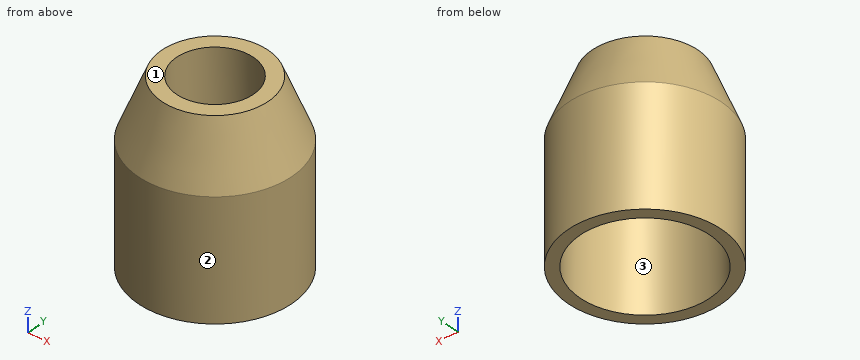
```python
from build123d import *

# Parameters (mm, degrees)
SKETCH177_R     = 6.5
PAD072_DEPTH    = 20
SKETCH178_R     = 3.25
POCKET069_DEPTH = 20.001
SKETCH179_R     = 5.5
POCKET070_DEPTH = 15
SKETCH180_W     = 0.76168
SKETCH180_H     = 6.5
PAD073_DEPTH    = 2
SKETCH182_W     = 6.5
SKETCH182_H     = 2
POCKET071_DEPTH = 6.501
SKETCH183_R     = 7.331051
POCKET072_DEPTH = 5


with BuildPart() as part:
    # Sketch177 → Pad072 (new body)
    with BuildSketch(Plane.XY):
        Circle(SKETCH177_R)
    extrude(amount=PAD072_DEPTH)

    # Sketch178 (on Face3 of Pad072) → Pocket069 (cut, through all)
    with BuildSketch(Plane.XY.offset(20)):
        Circle(SKETCH178_R)
    extrude(amount=-POCKET069_DEPTH, mode=Mode.SUBTRACT)

    # Sketch179 (on Face2 of Pocket069) → Pocket070 (cut)
    with BuildSketch(Plane(origin=(0, 0, 0), x_dir=(1, 0, 0), z_dir=(0, 0, -1))):
        Circle(SKETCH179_R)
    extrude(amount=-POCKET070_DEPTH, mode=Mode.SUBTRACT)

    # Sketch180 (on Face3 of Pocket070) → Pad073 (join)
    with BuildSketch(Plane.XY.offset(20)):
        with Locations((0.38084, -3.25)):
            Rectangle(SKETCH180_W, SKETCH180_H)
    extrude(amount=PAD073_DEPTH)

    # Sketch181 (on Face9 of Pad073) → Groove001 (revolve, cut)
    with BuildSketch(Plane(origin=(0, 0, 0), x_dir=(0, -1, 0), z_dir=(-1, 0, 0))):
        Polygon((4.5, 20), (6.5, 20), (6.5, 15), align=None)
    revolve(axis=Axis((0, 0, 0), (0, 0, 1)), mode=Mode.SUBTRACT)

    # Sketch182 (on Face9 of Groove001) → Pocket071 (cut, through all)
    with BuildSketch(Plane(origin=(0, 0, 0), x_dir=(0, -1, 0), z_dir=(-1, 0, 0))):
        with Locations((3.25, 21)):
            Rectangle(SKETCH182_W, SKETCH182_H)
    extrude(amount=-POCKET071_DEPTH, mode=Mode.SUBTRACT)

    # Sketch183 (on Face1 of Pocket071) → Pocket072 (cut)
    with BuildSketch(Plane(origin=(0, 0, 0), x_dir=(1, 0, 0), z_dir=(0, 0, -1))):
        Circle(SKETCH183_R)
    extrude(amount=-POCKET072_DEPTH, mode=Mode.SUBTRACT)


solid = part.part
```
Geometry: final body of the model. Coordinates: model frame, mm. Face numbers are marked on the shaded views. Give positions to 0.01 mm unless a question says otherwise; leave off trailing zeros. Loops run counter-clockwise (first coordinate to the right, second up) from the corner with the lowest first, then second, coordinate; pieces in that order, holes last. Notation, with made-up numbers: (-15.75, 24) -> (26.25, 24) arc R21 ccw to (26.25, 47) -> close; hole circle Ø8 at (-39, -1.75). An arc over 180 degrees is marked (long way). Return JSON: item names as keys, results as strings.
Item 1: Section A-A, the plane y = 0. Output: boundary loops of the cut face in (x, z), plus the area to 3 significant figures.
Filled in:
{"outline": "(-6.5, 5) -> (-5.5, 5) -> (-5.5, 15) -> (-3.25, 15) -> (-3.25, 20) -> (-4.5, 20) -> (-6.5, 15) -> close; (3.25, 15) -> (5.5, 15) -> (5.5, 5) -> (6.5, 5) -> (6.5, 15) -> (4.5, 20) -> (3.25, 20) -> close", "area": "42.5 mm^2"}
Item 2: Pin query (flat end, axial travel): P1, Ø2, axis at x = 2.5, y = 4, coming from the -Z side; P2, Ø2, axis at y = 2.5, z = 15.5, coming from the +X side; P3, Ø4, axis at x = 0, y = 0, coming from the -Z side; P4, Ø2, axis at y = 0.5, z = 16, coming from the +X side. Return the tip coordinate at first contact, or that it passes through.
Filled in:
{"P1": "z = 5", "P2": "x = 6.29", "P3": "through", "P4": "x = 6.49"}
Item 3: Section D-D, the plane z = 14.75. Output: boundary loops of the cut face in (x, y).
Filled in:
{"outline": "circle Ø13 at (0, 0); hole circle Ø11 at (0, 0)"}
Item 4: Line query: line 1 (Y direction, x = 0, z = 11.75); line 2 (X direction, y = 4, z = 13.75). Output: solid intervals per line, ascending.
Filled in:
{"line 1": "-6.5 to -5.5, 5.5 to 6.5", "line 2": "-5.12 to -3.77, 3.77 to 5.12"}
Item 5: Section C-C, the plane z = 16.75. Output: boundary loops of the cut face in (x, y).
Filled in:
{"outline": "circle Ø11.6 at (0, 0); hole circle Ø6.5 at (0, 0)"}
Item 6: Mould query, pull axis X, two halves, no side actions, for the marked faces 1, 2 and 3. Classes: released by +X, released by -X, zero draft, split by the parting line, or undercut.
Filled in:
{"face 1": "zero draft", "face 2": "split by the parting line", "face 3": "undercut"}
